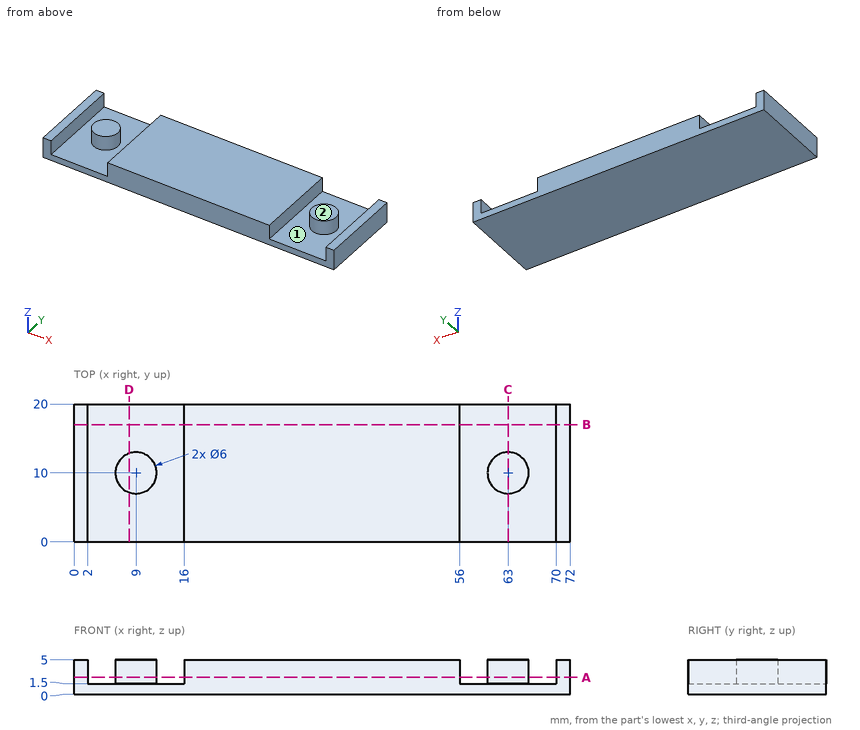
Source: three-view drawing plus pictorial views. Frame: mm from the lowest corner of the part. A direction names the side the tool comes from. Coordinates: 2 decimals unless noted, no trailing zeros. Loops run counter-clockwise (first coordinate to the right, second up) from the corner with the lowest first, then second, coordinate; pieces in that order, holes last. Notation, with made-up numbers: (-25, 26) - (13, 26) arc R26 ccw to (13, 53) - close; hole circle Ø4 at (-36, 52). An arc over 180 degrees is marked (long way). Answer in a Markdown table with one row per item. Add a question column.
Item 1: Section query D-D on x = 8. Return the cut outline in (y, z), then the cut area to 3 significant figures.
Item 2: Access query for the marked faces 1 and 2. Directions: +Z, -Z, +X, -X, +Y, -Y. A direction counts if a zero-diameter tool reaches every point of the face in a straight line with its end or side. Return the directions, or none.
Item 3: Section query C-C on x = 63. Return the cut outline in (y, z), then the cut area to 3 significant figures.
Item 4: Section query A-A on z = 2.45. Return the cut outline in (x, y), then the cut area to 3 significant figures.
Item 5: Line query: line 1 along X through (y, z) = (18, 4.05); line 2 along X through (y, z) = (10.25, 2.3); line 3 along X through (y, z) = (11, 4.7). Output: solid intervals per line, ascending. Write a range as [from, to].
Item 6: Section query B-B on y = 17. Return the cut outline in (x, z), then the cut area to 3 significant figures.
Recorded:
| question | item | result |
|---|---|---|
| 1 | outline | (0, 0) - (20, 0) - (20, 1.5) - (12.83, 1.5) - (12.83, 5) - (7.17, 5) - (7.17, 1.5) - (0, 1.5) - close |
| 1 | area | 49.8 mm^2 |
| 2 | face 1 | +Z |
| 2 | face 2 | +Z, +X, -X, +Y, -Y |
| 3 | outline | (0, 0) - (20, 0) - (20, 1.5) - (13, 1.5) - (13, 5) - (7, 5) - (7, 1.5) - (0, 1.5) - close |
| 3 | area | 51.0 mm^2 |
| 4 | outline | (0, 0) - (2, 0) - (2, 20) - (0, 20) - close; circle Ø6 at (9, 10); (16, 0) - (56, 0) - (56, 20) - (16, 20) - close; circle Ø6 at (63, 10); (70, 0) - (72, 0) - (72, 20) - (70, 20) - close |
| 4 | area | 937 mm^2 |
| 5 | line 1 | [0, 2], [16, 56], [70, 72] |
| 5 | line 2 | [0, 2], [6.01, 11.99], [16, 56], [60.01, 65.99], [70, 72] |
| 5 | line 3 | [0, 2], [6.17, 11.83], [16, 56], [60.17, 65.83], [70, 72] |
| 6 | outline | (0, 0) - (72, 0) - (72, 5) - (70, 5) - (70, 1.5) - (56, 1.5) - (56, 5) - (16, 5) - (16, 1.5) - (2, 1.5) - (2, 5) - (0, 5) - close |
| 6 | area | 262 mm^2 |
